Design review of the part built by this model. Coordinates are the model's own, in mm. Coordinates: 2 decimals unless noted, no trailing zeros. Write each loop counter-clockwise with the first axis right and the second up, starting at its lowest first coordinate (ties: lowest second). Pieces come first, ordered by that corner, then holes.
Q1. Take a section at A-A (x = 44). Give the boundary of the cut face in (y, z), and give its area (4 significant figures).
Q2. For probe 1 along Y at (x, z) = (99, 38.5); probe 2 along Z at (x, y) = (11.5, -3.5); probe 3 along Z at (x, y) = (58, 0.75), list the stretches that pass through material, from the lowest coordinate up.
Q3. Take a section at B-B (z = -78). Give the boundary of the cut face in (x, y).
Q4. Take a section at C-C (y = -5). Give the boundary of the cut face in (x, z), and give its area (3 significant figures).
Q5. Insertion check: pin 1 (8 mm diameter, centred on x = 76, z = 107, fed in from -Y); pin 2 (2.5 mm diameter, centred on x = 49, y = -3.5, fed in from -Z); pin 3 (0.8 mm diameter, centred on x = -87.5, z = 122.5, fed in from -Y). Each pin has a flat end and moves straight along its axis. Give the tip position at first contact, or say it passes through.
```python
from build123d import *

# Parameters (mm, degrees)
SKETCH1_W           = 268
SKETCH1_H           = 246
BOSS_EXTRUDE1_DEPTH = 1.5
BOSS_EXTRUDE2_DEPTH = 1.5
SWEEP1_PROFILE_R    = 1.75


with BuildPart() as part:
    # Sketch1 → Boss-Extrude1 (new body)
    with BuildSketch(Plane(origin=(0, 0, 0), x_dir=(1, 0, 0), z_dir=(0, 1, 0))):
        Rectangle(SKETCH1_W, SKETCH1_H)
    extrude(amount=BOSS_EXTRUDE1_DEPTH)

    # Sketch2 → Boss-Extrude2 (add)
    with BuildSketch(Plane.XY.offset(123)):
        Polygon((-134, 0), (134, 0), (134, -3), (12.5, -3), (12.5, -8), (-12.5, -8), (-12.5, -3), (-134, -3), align=None)
    extrude(amount=-BOSS_EXTRUDE2_DEPTH)

    # Sweep1: sweep along a path in Sketch3
    with BuildLine(Plane(origin=(0, 0, 0), x_dir=(1, 0, 0), z_dir=(0, 1, 0))) as sweep1_path:
        Line((-16, -123), (-16, -143))
        ThreePointArc((-16, -143), (-14.535533906, -146.535533906), (-11, -148))
        Line((-11, -148), (11, -148))
        ThreePointArc((11, -148), (14.535533906, -146.535533906), (16, -143))
        Line((16, -143), (16, -123))
    # Sweep1 profile (on start of the path) → Sweep1 (sweep)
    with BuildSketch(Plane(origin=(-16, 0, 123), x_dir=(1, 0, 0), z_dir=(0, 0, 1))):
        Circle(SWEEP1_PROFILE_R)
    sweep(path=sweep1_path.line)


solid = part.part
```
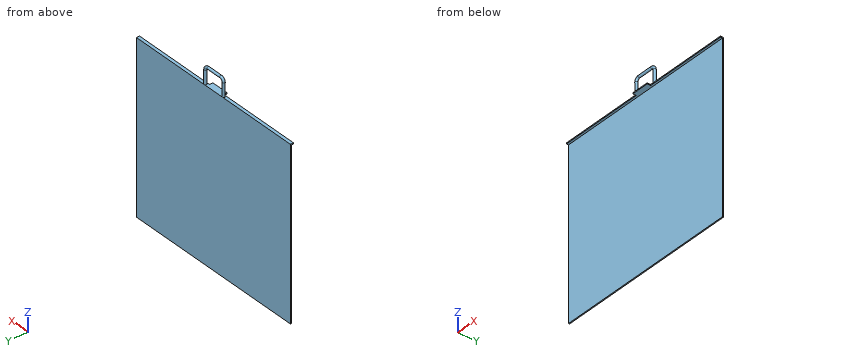
Response:
1. outline: (-3, 121.5) - (0, 121.5) - (0, -123) - (1.5, -123) - (1.5, 123) - (-3, 123) - close
1. area: 373.5 mm2
2. probe 1: y = 0 to 1.5
2. probe 2: z = 121.5 to 123
2. probe 3: z = -123 to 123
3. outline: (-134, 0) - (134, 0) - (134, 1.5) - (-134, 1.5) - close
4. outline: (-12.5, 121.5) - (12.5, 121.5) - (12.5, 123) - (-12.5, 123) - close
4. area: 37.5 mm2
5. pin 1: stops at y = 0
5. pin 2: stops at z = 121.5
5. pin 3: stops at y = -3
